Here's the drawing with two shaded views (mm, measured from the low corner). I have some questions. Give positions to 0.01 mm unless a question says otherwise; leave off trailing zeros. Loops run counter-clockwise (first coordinate to the right, second up) from the corner with the lowest first, then second, coordinate; pieces in that order, holes last. Notation, with made-up numbers: (35, 37) - (40, 37) arc R19 cw to (40, 52) - close; hole circle Ø10 at (63, 36.25). An arc over 180 degrees is marked (long way). Answer as a JSON object with one key per item and string values. Group by question number.
Item 1: Will these pins go through, and if not, where does the flat tip stop? pin 1 (6 mm diameter, centred on x = 21, z = 14, fed in from +Y); pin 2 (1 mm diameter, centred on x = 42, z = 39.5, fed in from +Y); pin 3 (2 mm diameter, centred on y = 6, z = 31, fed in from +X).
Item 2: Suppose I cut it at A-A on x = 10. Write out the boundary of the cut face in (y, z), and give its area (3 significant figures).
Item 3: Thinking about a two-plate mould opening in X: for the marked faces 1 and 2, which applies, pulls with the +X half, pulls with the -X half, needs draft (parallel to the pull), parting line crosses it, or undercut?
Item 4: Suppose I cut it at C-C on x = 57. Write out the boundary of the cut face in (y, z), and give its area (3 significant figures).
Item 5: Suppose I cut it at D-D on y = 6.75. Write out the boundary of the cut face in (x, z).
Item 6: Please list where these lines run through material, in increasing order: L1, parallel to X at y = 1.85, z = 22; L2, parallel to X at y = 2.75, z = 26; L3, parallel to Y at x = 68.5, z = 2.5.
Item 7: Suppose I cut it at B-B on z = 13. Write out the boundary of the cut face in (x, y).
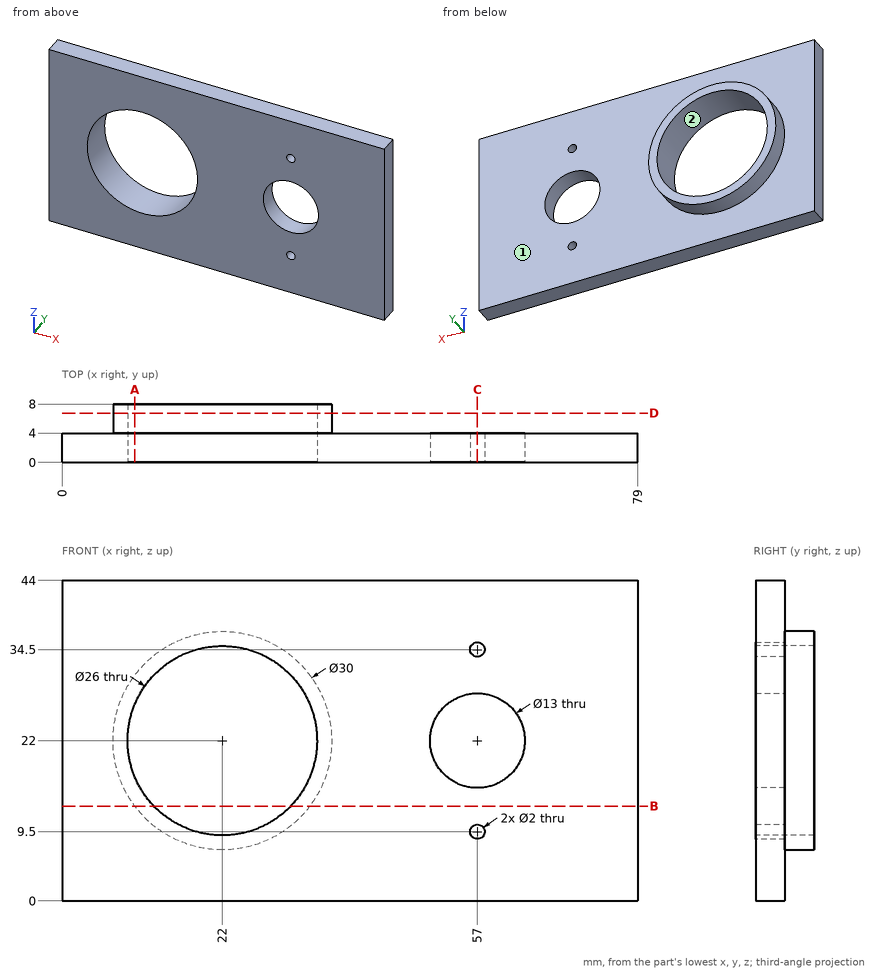
Worked out:
{
 "1": {"pin 1": "passes through", "pin 2": "stops at y = 4", "pin 3": "stops at x = 34.69"},
 "2": {"outline": "(0, 0) - (4, 0) - (4, 13) - (8, 13) - (8, 17) - (0, 17) - close; (0, 27) - (8, 27) - (8, 31) - (4, 31) - (4, 44) - (0, 44) - close", "area": "168 mm2"},
 "3": {"face 1": "needs draft", "face 2": "undercut"},
 "4": {"outline": "(0, 0) - (4, 0) - (4, 8.5) - (0, 8.5) - close; (0, 10.5) - (4, 10.5) - (4, 15.5) - (0, 15.5) - close; (0, 28.5) - (4, 28.5) - (4, 33.5) - (0, 33.5) - close; (0, 35.5) - (4, 35.5) - (4, 44) - (0, 44) - close", "area": "108 mm2"},
 "5": {"outline": "circle Ø30 at (22, 22); hole circle Ø26 at (22, 22)"},
 "6": {"L1": "x = 0 to 9, 35 to 50.5, 63.5 to 79", "L2": "x = 0 to 9.63, 34.37 to 51.88, 62.12 to 79", "L3": "y = 0 to 4"},
 "7": {"outline": "(0, 0) - (12.62, 0) - (12.62, 8) - (10, 8) - (10, 4) - (0, 4) - close; (31.38, 0) - (79, 0) - (79, 4) - (34, 4) - (34, 8) - (31.38, 8) - close"}
}
